CAD build for the part. Positions are in the model's coordinates, mm. Face numbers are marked on the shaded views. A direction names the side the tool comes from. Give positions to 0.01 mm unless a question says otherwise; leave off trailing zeros. Write each loop counter-clockwise with the first axis right and the second up, starting at its lowest first coordinate (ties: lowest second). Pieces come first, ordered by that corner, then holes. Notation, with made-up numbers: (45.5, -10.5) - (50.5, -10.5) arc R29 cw to (50.5, 22.5) - close; hole circle Ø11 at (23, 24). An arc over 180 degrees is marked (long way). Put each result on its own line as item: value. Start each with the question number.
1. Drop flat-ended pins along their axis: pin 1 (3.5 mm diameter, centred on y = 106.5, z = 0.5, fed in from +X) (3 decimals); pin 2 (1 mm diameter, centred on x = 6.5, z = 2, fed in from -Y); pin 3 (1 mm diameter, centred on x = 4, y = 106, fed in from +Z); pin 4 (5 mm diameter, centred on y = 104.775, z = 0, fed in from -X). Give the stop position or say it passes through.
2. Cut at C-C on x = 7.5. List the corners of the cut face in (y, z), and give its area (3 significant figures).
3. Wall check: line 1 (Y direction, x = -0.05, z = 0); line 2 (Z direction, x = -2, y = 109.5); line 3 (X direction, y = 112.5, z = 0.25) (3 decimals). Give the ranges that are in metal, low to high.
4. Tool access for the marked faces 1, 2 and 3: list every direction of +Z, -Z, +X, -X, +Y, -Y with a clear straight run to the whole face (end or side of a thin tool).
Autodesk Inventor part; units mm, degrees
ref_plane "YZ Plane" through (0, 0, 0) normal (1, 0, 0) x (0, 1, 0)
ref_plane "XZ Plane" through (0, 0, 0) normal (0, 1, 0) x (-1, 0, 0)
ref_plane "XY Plane" through (0, 0, 0) normal (0, 0, 1) x (1, 0, 0)
sketch "Sketch1" plane through (0, 0, 0) normal (0, 1, 0) x (-1, 0, 0)
  line L0 (3.175, -4.7625) -> (-3.175, -4.7625)
  line L1 (-3.175, -4.7625) -> (-3.175, 4.7625)
  line L2 (-3.175, 4.7625) -> (3.175, 4.7625)
  line L3 (3.175, 4.7625) -> (3.175, -4.7625)
  line L4 (3.175, -4.7625) -> (-3.175, 4.7625) construction
  line L5 (-3.175, -4.7625) -> (3.175, 4.7625) construction
  point P0 (0, 0)
  point P1 (0, 0)
  point P2 (0, 0)
  point P3 (0, 0)
  dimension "d0" = 9.525
  dimension "d1" = 6.35
extrude "Extrusion1" add sketch "Sketch1" along normal blind 120.65
sketch "Sketch2" plane through (0, 0, 0) normal (0, -1, 0) x (1, 0, 0)
  line L0 (3.175, 4.7625) -> (12.7, 4.7625)
  line L1 (12.7, 4.7625) -> (12.7, -4.7625)
  line L2 (12.7, -4.7625) -> (3.175, -4.7625)
  line L3 (3.175, -4.7625) -> (3.175, 4.7625)
  point P0 (0, 0)
  dimension "d4" = 9.525
extrude "Extrusion2" add sketch "Sketch2" against normal blind 4.7625
sketch "Sketch3" plane through (0, 120.65, 0) normal (0, 1, 0) x (1, 0, 0)
  line L0 (3.175, -4.7625) -> (3.175, 4.7625)
  line L1 (3.175, -4.7625) -> (12.7, -4.7625)
  line L2 (12.7, -4.7625) -> (12.7, 4.7625)
  line L3 (12.7, 4.7625) -> (3.175, 4.7625)
  point P0 (0, 0)
extrude "Extrusion3" add sketch "Sketch3" against normal blind 4.7625
fillet "Fillet1" radius 3.175 4 edges at (12.7, 2.3813, -4.7625) (12.7, 2.3813, 4.7625) (12.7, 118.2687, -4.7625) (12.7, 118.2687, 4.7625)
fillet "Fillet2" radius 3.175 2 edges at (3.175, 4.7625, 0) (3.175, 115.8875, 0)
fillet "Fillet3" radius 1.27 12 edges at (7.9375, 115.8875, -4.7625) (11.7701, 115.8875, -3.8326) (12.7, 115.8875, 0) (11.7701, 115.8875, 3.8326) (7.9375, 115.8875, 4.7625) (3.175, 60.325, 4.7625) (7.9375, 4.7625, 4.7625) (11.7701, 4.7625, 3.8326) (12.7, 4.7625, 0) (11.7701, 4.7625, -3.8326) (7.9375, 4.7625, -4.7625) (3.175, 60.325, -4.7625)
sketch "Sketch7" plane through (3.175, 7.9375, 3.4925) normal (1, 0, 0) x (0, 0, -1)
  line L0 (0, 0) -> (0, 104.775)
  line L1 (5.08, -7.9375) -> (1.905, -7.9375)
  line L2 (0, 52.3875) -> (19.363, 52.3875)
  point P0 (3.4925, -7.9375)
  point P1 (3.4925, 7.9375)
  point P2 (3.4925, 30.1625)
  point P3 (3.4925, 52.3875)
  point P4 (3.4925, 96.8375)
  point P5 (3.4925, 74.6125)
  point P6 (3.4925, 19.05)
  point P7 (3.4925, 41.275)
  point P8 (3.4925, 85.725)
  point P9 (3.4925, 63.5)
  dimension "d25" = 15.875
  dimension "d26" = 22.225
  dimension "d27" = 11.1125
  dimension "d28" = 11.1125
hole "Hole2" at (3.175, 15.875, 0) at (3.175, 38.1, 0) at (3.175, 60.325, 0) at (3.175, 82.55, 0) at (3.175, 104.775, 0) at (3.175, 26.9875, 0) at (3.175, 49.2125, 0) at (3.175, 93.6625, 0) at (3.175, 71.4375, 0) direction (-1, 0, 0) diameter 3.175 depth 203.2 tip angle 118
fillet "Fillet4" radius 1.27 9 edges at (3.175, 104.775, 1.5875) (3.175, 93.6625, 1.5875) (3.175, 82.55, 1.5875) (3.175, 71.4375, 1.5875) (3.175, 60.325, 1.5875) (3.175, 49.2125, 1.5875) (3.175, 38.1, 1.5875) (3.175, 26.9875, 1.5875) (3.175, 15.875, 1.5875)
fillet "Fillet5" radius 1.27 9 edges at (-3.175, 104.775, 1.5875) (-3.175, 93.6625, 1.5875) (-3.175, 82.55, 1.5875) (-3.175, 71.4375, 1.5875) (-3.175, 60.325, 1.5875) (-3.175, 49.2125, 1.5875) (-3.175, 38.1, 1.5875) (-3.175, 26.9875, 1.5875) (-3.175, 15.875, 1.5875)
fillet "Fillet6" radius 1.27 2 edges at (-3.175, 60.325, -4.7625) (-3.175, 60.325, 4.7625)
sketch "Sketch4" plane through (0, 120.65, 0) normal (0, 1, 0) x (1, 0, 0)
  line L0 (12.7, -1.5875) -> (12.7, 1.5875)
  point P0 (0, 0)
  point P1 (7.62, 0)
  point P2 (12.7, 0)
  dimension "d11" = 5.08
ref_plane "Work Plane3" through (0, 95.25, 0) normal (0, 1, 0) x (1, 0, 0)
sketch "Sketch11" plane through (0, 95.25, 0) normal (0, 1, 0) x (1, 0, 0)
  line L0 (-3.175, 4.7625) -> (12.7, 4.7625)
  line L1 (12.7, 4.7625) -> (12.7, -4.7625)
  line L2 (12.7, -4.7625) -> (-3.175, -4.7625)
  line L3 (-3.175, -4.7625) -> (-3.175, 4.7625)
  arc A0 (-3.175, -3.4925) -> (-1.905, -4.7625) centre (-1.905, -3.4925) ccw
  line L4 (-3.175, -3.4925) -> (-3.175, 3.4925)
  arc A1 (-1.905, 4.7625) -> (-3.175, 3.4925) centre (-1.905, 3.4925) ccw
  line L5 (-1.905, 4.7625) -> (9.525, 4.7625)
  arc A2 (12.7, 1.5875) -> (9.525, 4.7625) centre (9.525, 1.5875) ccw
  line L6 (12.7, 1.5875) -> (12.7, -1.5875)
  arc A3 (9.525, -4.7625) -> (12.7, -1.5875) centre (9.525, -1.5875) ccw
  line L7 (9.525, -4.7625) -> (-1.905, -4.7625)
  point P0 (0, 0)
extrude "Extrusion10" cut sketch "Sketch11" against normal through all contours L0 A2 L1 A3 L2 A0 L3 A1
properties part number "LidSupportLW"
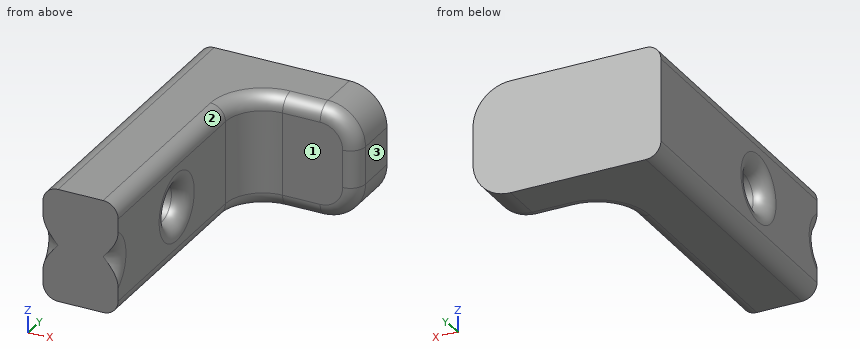
Report:
1. pin 1: stops at x = 3.175
1. pin 2: stops at y = 115.87
1. pin 3: passes through
1. pin 4: stops at x = -3.12
2. outline: (115.89, -3.49) arc R1.27 ccw to (117.16, -4.76) - (120.65, -4.76) - (120.65, 4.76) - (117.16, 4.76) arc R1.27 ccw to (115.89, 3.49) - close
2. area: 44.7 mm²
3. line 1: y = 95.25 to 103.19, 106.36 to 120.65
3. line 2: z = -4.76 to 4.76
3. line 3: x = -3.175 to 3.175
4. face 1: +Z, -Z, +X, -Y
4. face 2: +Z, +X, -Y
4. face 3: +Z, -Z, +X, +Y, -Y
